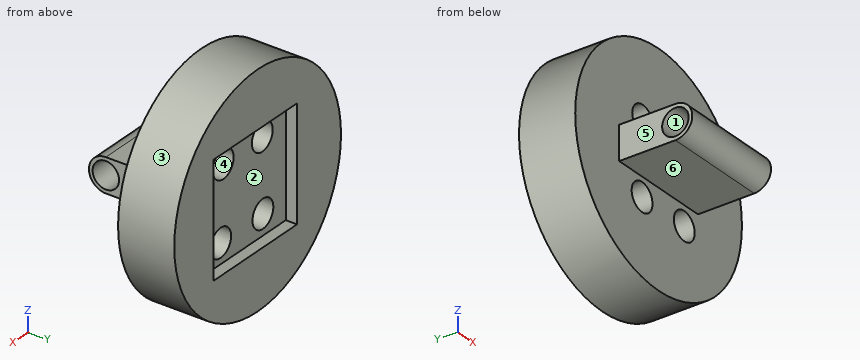
Autodesk Inventor part; units mm, degrees
ref_plane "YZ Plane" through (0, 0, 0) normal (1, 0, 0) x (0, 1, 0)
ref_plane "XZ Plane" through (0, 0, 0) normal (0, 1, 0) x (-1, 0, 0)
ref_plane "XY Plane" through (0, 0, 0) normal (0, 0, 1) x (1, 0, 0)
sketch "Sketch1" plane through (0, 0, 0) normal (1, 0, 0) x (0, 1, 0)
  circle A0 centre (0, 0) radius 2.9972
  arc A1 (0, 3.81) -> (0, -3.81) centre (0, 0) ccw
  line L0 (0, 3.81) -> (12.7, 3.81)
  line L1 (0, -3.81) -> (12.7, -3.81)
  line L2 (12.7, -3.81) -> (12.7, 3.81)
  dimension "d0" = 5.9944
  dimension "d4" = 7.62
  dimension "d5" = 12.7
  dimension "d6" = 12.7
extrude "Extrusion1" add sketch "Sketch1" along normal blind 24.003
sketch "Sketch2" plane through (0, 12.7, 3.81) normal (0, 1, 0) x (1, 0, 0)
  line L0 (0, 7.62) -> (24.003, 7.62)
  circle A0 centre (12.0015, 3.81) radius 25.4
  point P0 (0, 3.81)
  dimension "d9" = 50.8
extrude "Extrusion2" add sketch "Sketch2" along normal blind 12.7
sketch "Sketch3" plane through (12.0015, 25.4, 0) normal (0, 1, 0) x (1, 0, 0)
  line L0 (-12.0015, 2.9972) -> (-12.0015, -2.9972)
  line L1 (-12.0015, -12.7) -> (-12.0015, 12.7)
  line L2 (-12.0015, -12.7) -> (13.3985, -12.7)
  line L3 (13.3985, -12.7) -> (13.3985, 12.7)
  line L4 (13.3985, 12.7) -> (-12.0015, 12.7)
  line L5 (-12.0015, 12.7) -> (-12.0015, -12.7)
  circle A0 centre (-5.6515, -8.128) radius 1.905
  line L6 (13.3985, -12.7) -> (13.3985, -8.128)
  line L7 (13.3985, -12.7) -> (13.3985, -8.128)
  line L8 (13.3985, -12.7) -> (13.3985, -8.128)
  circle A1 centre (7.0485, -8.128) radius 1.905
  circle A2 centre (-5.6515, 8.128) radius 1.905
  circle A3 centre (7.0485, 8.128) radius 1.905
  circle A4 centre (-5.6515, -8.128) radius 1.905
  circle A5 centre (7.0485, -8.128) radius 1.905
  point P0 (-12.0015, 0)
  dimension "d13" = 25.4
  dimension "d14" = 25.4
  dimension "d17" = 3.81
  dimension "d20" = 3.81
  dimension "d23" = 3.81
  dimension "d24" = 3.81
  dimension "d25" = 3.81
  dimension "d26" = 3.81
extrude "Extrusion3" cut sketch "Sketch3" against normal blind 2.54
sketch "Sketch4" plane through (6.35, 25.4, 8.128) normal (0, 1, 0) x (1, 0, 0)
  point P0 (-6.35, 8.128)
  point P1 (0.8022, -0.041)
hole "Hole1" at (7.1522, 25.4, 8.169) direction (0, -1, 0) diameter 6.35 end through all
sketch "Sketch5" plane through (6.35, 25.4, -8.128) normal (0, 1, 0) x (1, 0, 0)
  point P0 (-6.35, -8.128)
  point P1 (0.6252, -0.0267)
  point P2 (13.4879, 0.0841)
  point P3 (12.7137, -16.0745)
hole "Hole2" at (6.9752, 25.4, -8.1013) at (19.8379, 25.4, -8.2121) at (19.0637, 25.4, 7.9465) direction (0, -1, 0) diameter 6.35 end through all
properties part number "shaft_mount_wrist"
Geometry: final body of the model. Coordinates: model frame, mm. Face numbers are marked on the shaded views. A direction names the side the tool comes from. Round coordinates to 2 decimals unless told otherwise and drop trailing zeros. Loops run counter-clockwise (first coordinate to the right, second up) from the corner with the lowest first, then second, coordinate; pieces in that order, holes last. Notation, with made-up numbers: M -2.5,55 L 39.5,55 A16 ccw 39.5,79 Z; hole C 77.25,53.5 d5. An arc over 180 degrees is marked long. Put each result on its own line as item: value. Start each with the question number.
(1) Section query B-B (y = 21.75). State how many separate pieces and enclosed holes the cut face has, then the cut area to 3 significant figures.
(2) Section query A-A (z = 0). Return loops of the section in (x, y).
(3) Material intervals for line 1 along Z through (x, y) = (19, 0); line 2 along Z through (x, y) = (17, 18); line 3 along Y through (x, z) = (14.5, 9), sorted ascending. Write a range as [from, to].
(4) Section query D-D (y = 11.5). Return loops of the section in (x, z), then the cut area to 3 significant figures.
(5) Section query C-C (z = 10.5). Return loops of the section in (x, y).
(6) Contact query for flat-ended pins moving along their axis: pin 1 Ø7.5 at (x, z) = (15.5, -3) entering from +Y; pin 2 Ø2 at (x, y) = (13, 24) entering from +Z; pin 3 Ø1.3 at (y, z) = (23.5, 2) entering from +X; pin 4 Ø10 at (x, z) = (19.84, -8.21) entering from +Y. Output: stop coordinate, or through.
(7) Draft query along X for the marked faces 1, 2 and 3. Return one class per face: +X half, -X half, draft (parallel to the pull), parting line (faces both ways), or undercut.
(8) Set-up query: the marked faces 4, 5 and 6. Return all of +Z, -Z, +X, -X, +Y, -Y with unobstructed straight access to the full face (end or side cutting, diameter ignored); none if empty.
Findings below:
1. separate pieces: 1
1. enclosed holes: 4
1. area: 1,900 mm2
2. outline: M -13.4,12.7 L 0,12.7 L 0,3 L 24,3 L 24,12.7 L 37.4,12.7 L 37.4,25.4 L 25.4,25.4 L 25.4,22.86 L 0,22.86 L 0,25.4 L -13.4,25.4 Z; M 0,-3.81 L 24,-3.81 L 24,-3 L 0,-3 Z
3. line 1: z = [-3.81, -3], [3, 3.81]
3. line 2: z = [-24.9, -9.64], [-6.79, 5.53], [10.36, 24.9]
3. line 3: y = [12.7, 22.86]
4. outline: M 0,-3.81 L 24,-3.81 L 24,3.81 L 0,3.81 Z
4. area: 183 mm2
5. outline: M -11.13,12.7 L 5,12.7 L 5,22.86 L 0,22.86 L 0,25.4 L -11.13,25.4 Z; M 9.31,12.7 L 17.18,12.7 L 17.18,22.86 L 9.31,22.86 Z; M 20.95,12.7 L 35.13,12.7 L 35.13,25.4 L 25.4,25.4 L 25.4,22.86 L 20.95,22.86 Z
6. pin 1: stops at y = 22.86
6. pin 2: stops at z = 25.4
6. pin 3: stops at x = 37.37
6. pin 4: stops at y = 25.4
7. face 1: draft
7. face 2: undercut
7. face 3: parting line
8. face 4: +Y, -Y
8. face 5: +Z, -Z, -X, -Y
8. face 6: -Z, +X, -X, -Y
